from build123d import *

# Parameters (mm, degrees)
SKETCH1_R           = 3.2
SKETCH1_R_2         = 14
BOSS_EXTRUDE1_DEPTH = 6.35
SKETCH2_R           = 1.5
CUT_EXTRUDE1_DEPTH  = 736.05148275


with BuildPart() as part:
    # Sketch1 → Boss-Extrude1 (new body)
    with BuildSketch(Plane.XY):
        Polygon((-647.460250444, -317.619540534), (-477.475995614, -23.198174681), (-442.475995614, -23.198174681), (-272.491740783, -317.619540534), (-289.991740783, -347.930429667), (-629.960250444, -347.930429667), align=None)
        with Locations((-581.209182953, -222.869325584)):
            Circle(SKETCH1_R, mode=Mode.SUBTRACT)
        with Locations((-528.649182953, -131.832735139)):
            Circle(SKETCH1_R, mode=Mode.SUBTRACT)
        with Locations((-500.577727615, -148.011529753)):
            Circle(SKETCH1_R, mode=Mode.SUBTRACT)
        with Locations((-553.136815613, -239.046537702)):
            Circle(SKETCH1_R, mode=Mode.SUBTRACT)
        with Locations((-367.294158494, -238.209054553)):
            Circle(SKETCH1_R, mode=Mode.SUBTRACT)
        with Locations((-419.854158494, -147.172464107)):
            Circle(SKETCH1_R, mode=Mode.SUBTRACT)
        with Locations((-391.545684719, -131.412060795)):
            Circle(SKETCH1_R, mode=Mode.SUBTRACT)
        with Locations((-338.985684719, -222.448651241)):
            Circle(SKETCH1_R, mode=Mode.SUBTRACT)
        with Locations((-511.800751787, -305.530429667)):
            Circle(SKETCH1_R, mode=Mode.SUBTRACT)
        with Locations((-406.680508256, -305.530429667)):
            Circle(SKETCH1_R, mode=Mode.SUBTRACT)
        with Locations((-406.680630022, -337.930429667)):
            Circle(SKETCH1_R, mode=Mode.SUBTRACT)
        with Locations((-511.800630022, -337.930429667)):
            Circle(SKETCH1_R, mode=Mode.SUBTRACT)
        with Locations((-459.807870528, -114.054080446)):
            Circle(SKETCH1_R_2, mode=Mode.SUBTRACT)
        with Locations((-358.022290508, -290.351876517)):
            Circle(SKETCH1_R_2, mode=Mode.SUBTRACT)
        with Locations((-561.593450547, -290.351876517)):
            Circle(SKETCH1_R_2, mode=Mode.SUBTRACT)
        with BuildLine():
            Line((-425.750841471, -154.687649698), (-376.750841471, -239.558139269))
            ThreePointArc((-376.750841471, -239.558139269), (-379.734271663, -250.692452327), (-390.86858472, -247.709022135))
            Line((-390.86858472, -247.709022135), (-439.86858472, -162.838532564))
            ThreePointArc((-439.86858472, -162.838532564), (-436.885154528, -151.704219506), (-425.750841471, -154.687649698))
        make_face(mode=Mode.SUBTRACT)
        with BuildLine():
            Line((-410.240508256, -299.529344232), (-508.240508256, -299.529344232))
            ThreePointArc((-508.240508256, -299.529344232), (-516.391391121, -291.378461367), (-508.240508256, -283.227578501))
            Line((-508.240508256, -283.227578501), (-410.240508256, -283.227578501))
            ThreePointArc((-410.240508256, -283.227578501), (-402.089625391, -291.378461367), (-410.240508256, -299.529344232))
        make_face(mode=Mode.SUBTRACT)
        with BuildLine():
            Line((-543.432261857, -240.54083955), (-494.432261857, -155.67034998))
            ThreePointArc((-494.432261857, -155.67034998), (-483.297948799, -152.686919788), (-480.314518607, -163.821232845))
            Line((-480.314518607, -163.821232845), (-529.314518607, -248.691722416))
            ThreePointArc((-529.314518607, -248.691722416), (-540.448831665, -251.675152608), (-543.432261857, -240.54083955))
        make_face(mode=Mode.SUBTRACT)
    extrude(amount=BOSS_EXTRUDE1_DEPTH)

    # Sketch2 → Cut-Extrude1 (cut, through all)
    with BuildSketch(Plane.XY):
        with Locations((-451.975995614, -46.198174681)):
            Circle(SKETCH2_R)
        with Locations((-291.308942687, -336.211907881)):
            Circle(SKETCH2_R)
        with Locations((-467.975995614, -30.198174681)):
            Circle(SKETCH2_R)
        with Locations((-451.975995614, -30.198174681)):
            Circle(SKETCH2_R)
        with Locations((-467.975995614, -46.198174681)):
            Circle(SKETCH2_R)
        with Locations((-283.308957903, -322.355492635)):
            Circle(SKETCH2_R)
        with Locations((-297.163015743, -314.351426082)):
            Circle(SKETCH2_R)
        with Locations((-305.165363337, -328.211898695)):
            Circle(SKETCH2_R)
        with Locations((-614.791666157, -328.203188331)):
            Circle(SKETCH2_R)
        with Locations((-622.791666157, -314.34678187)):
            Circle(SKETCH2_R)
        with Locations((-628.648072618, -336.203188331)):
            Circle(SKETCH2_R)
        with Locations((-636.648072618, -322.34678187)):
            Circle(SKETCH2_R)
    extrude(amount=CUT_EXTRUDE1_DEPTH, mode=Mode.SUBTRACT)


solid = part.part
Verification items for the finished model (mm, model axes). A direction names the side the tool comes from. Give positions to 0.01 mm unless a question says otherwise; leave off trailing zeros. Loops run counter-clockwise (first coordinate to the right, second up) from the corner with the lowest first, then second, coordinate; pieces in that order, holes last. Notation, with made-up numbers: (57, 6) - (102, 6) arc R17 ccw to (102, 11) - close; hole circle Ø8 at (36.25, 77.5). An arc over 180 degrees is marked (long way). Write item = value, one per line. Start each with the question number.
Q1. Tool access check on faces 4 (the face through (-563.66, -172.47, 3.13)), 5 (the face through (-516.39, -291.56, 3.13)). Record the directions out of +Z, -Z, +X, -X, +Y, -Y that give a thin tool (end or side, any length) a straight path to the whole face; none if there is none.
Q2. Cross-section at A-A, the plane y = -123. Enter the section's corners in (x, z), and give its area (3 significant figures).
Q3. Thickness scan on line 1 (X direction, y = -200, z = 1); line 2 (Y direction, x = -437.5, z = 3.75); line 3 (Y direction, x = -503.5, z = 5.25). Record the ranges inside material, lowest first.
Q4. Mould release check, pull along Y, two halves, no side actions. Record for faces 1 (the face through (-281.119, -332.563, 3.131)), 2 (the face through (-540.293, -251.763, 3.131)), 3 (the face through (-457, -219, 0)): released by +Y, released by -Y, zero draft, split by the parting line, or undercut.
Q5. Cross-section at C-C, the plane y = -295. Enter the section's corners in (x, z), and give its area (3 significant figures).
Q6. Cross-section at D-D, the plane z = 5. State how many separate pieces and enclosed holes the cut face has, and give its area (4 significant figures).
Q7. Cross-section at B-B, the plane x = -566. Enter the section's corners in (y, z), and give its area (3 significant figures).
Q8. Depth check by flat-ended pin: P1, Ø2, axis at y = -197.5, z = 1.5, coming from the -X side. Enter the tip coordinate at first touch or a pass-through.
Answer key:
q1.face_4 = +Z, -Z, -X, +Y
q1.face_5 = +Z, -Z
q2.outline = (-535.1, 0) - (-470.58, 0) - (-470.58, 6.35) - (-535.1, 6.35) - close; (-449.04, 0) - (-384.86, 0) - (-384.86, 6.35) - (-449.04, 6.35) - close
q2.area = 817 mm^2
q3.line_1 = -579.55 to -520.03, -501.2 to -418.41, -399.59 to -340.4
q3.line_2 = -347.93 to -299.53, -283.23 to -166.94, -152.1 to -31.82
q3.line_3 = -347.93 to -299.53, -283.23 to -203.98, -171.38 to -149.32, -146.71 to -68.27
q4.face_1 = released by -Y
q4.face_2 = undercut
q4.face_3 = zero draft
q5.outline = (-634.4, 0) - (-574.8, 0) - (-574.8, 6.35) - (-634.4, 6.35) - close; (-548.39, 0) - (-515.54, 0) - (-515.54, 6.35) - (-548.39, 6.35) - close; (-402.94, 0) - (-371.23, 0) - (-371.23, 6.35) - (-402.94, 6.35) - close; (-344.82, 0) - (-285.55, 0) - (-285.55, 6.35) - (-344.82, 6.35) - close
q5.area = 1,160 mm^2
q6.separate_pieces = 1
q6.enclosed_holes = 30
q6.area = 63,450 mm^2
q7.outline = (-347.93, 0) - (-303.64, 0) - (-303.64, 6.35) - (-347.93, 6.35) - close; (-277.06, 0) - (-176.53, 0) - (-176.53, 6.35) - (-277.06, 6.35) - close
q7.area = 920 mm^2
q8.P1 = -578.69
